```python
from build123d import *

# Parameters (mm, degrees)
F0_R         = 3.95
F0_R_2       = 2.95
F1_DEPTH     = 12
F3_DEPTH     = 4
F5_R         = 5
F6_W         = 3
F6_H         = 7
F6_W_2       = 2.1112600537
F7_DEPTH     = 16.5
F8_W         = 3.25
F8_H         = 1.5
F9_DEPTH     = 7
F10_T1_DEPTH = 34
F10_T3_DEPTH = 24.5


# Not quite as in the source:
# - a fillet or chamfer that OpenCascade refuses, or shapes differently, is made with other operations: its cross-section is extruded or revolved along the edge and cut away or added


with BuildPart() as f1:
    # F0 (on Top) → F1 (new body)
    with BuildSketch(Plane.XY):
        Circle(F0_R)
        Circle(F0_R_2, mode=Mode.SUBTRACT)
    extrude(amount=F1_DEPTH)


with BuildPart() as f1b:
    # F0 (on Top) → F1, piece 2 (new body)
    with BuildSketch(Plane.XY):
        with Locations((29.5, 0)):
            Circle(F0_R)
        with Locations((29.5, 0)):
            Circle(F0_R_2, mode=Mode.SUBTRACT)
    extrude(amount=F1_DEPTH)


with BuildPart() as f3:
    # F2 (on face) → F3 (new body)
    with BuildSketch(Plane(origin=(0, 0, 0), x_dir=(1, 0, 0), z_dir=(0, 0, -1))):
        with BuildLine():
            ThreePointArc((0, 3.95), (2.7930717857, 2.7930717857), (3.95, 0))
            Line((3.95, 0), (25.55, 0))
            ThreePointArc((25.55, 0), (26.7069282143, 2.7930717857), (29.5, 3.95))
            Line((29.5, 3.95), (29.5, 20))
            Line((29.5, 20), (0, 20))
            Line((0, 20), (0, 3.95))
        make_face()
    extrude(amount=-F3_DEPTH)

    # F4: union F1, F1b
    add(f1.part)
    add(f1b.part)

    # F5
    f5_edges = [f3.edges().sort_by_distance(p)[0] for p in [
        (0, -20, 2),
        (29.5, -20, 2),
    ]]
    fillet(f5_edges, radius=F5_R)

    # F6 (on face) → F7 (join)
    with BuildSketch(Plane(origin=(0, 0, 0), x_dir=(1, 0, 0), z_dir=(0, 0, -1))):
        with Locations((-3.6112600537, 11.5)):
            Rectangle(F6_W, F6_H)
        with Locations((-1.0556300269, 11.5)):
            Rectangle(F6_W_2, F6_H)
        with Locations((30.5556300269, 11.5)):
            Rectangle(F6_W_2, F6_H)
        with Locations((33.1112600537, 11.5)):
            Rectangle(F6_W, F6_H)
    extrude(amount=-F7_DEPTH)

    # F8 (on face) → F9 (cut, through all)
    with BuildSketch(Plane.XZ.offset(15)):
        with Locations((-1.625, 12.75)):
            Rectangle(F8_W, F8_H)
        with Locations((31.125, 12.75)):
            Rectangle(F8_W, F8_H)
    extrude(amount=-F9_DEPTH, mode=Mode.SUBTRACT)

    # F10: fillet of radius 3.5 on 6 edges, made by hand

    # F10_s2 → F10_t1 (cut)
    with BuildSketch(Plane.XY.offset(-8.75)):
        with BuildLine():
            ThreePointArc((-1.6112600537, -15), (-4.0861337879, -13.9748737342), (-5.1112600537, -11.5))
            Line((-5.1112600537, -11.5), (-5.1112600537, -15))
            Line((-5.1112600537, -15), (-1.6112600537, -15))
        make_face()
        with BuildLine():
            ThreePointArc((-5.1112600537, -11.5), (-4.0861337879, -9.0251262658), (-1.6112600537, -8))
            Line((-1.6112600537, -8), (-5.1112600537, -8))
            Line((-5.1112600537, -8), (-5.1112600537, -11.5))
        make_face()
        with BuildLine():
            ThreePointArc((34.6112600537, -11.5), (33.5861337879, -13.9748737342), (31.1112600537, -15))
            Line((31.1112600537, -15), (34.6112600537, -15))
            Line((34.6112600537, -15), (34.6112600537, -11.5))
        make_face()
        with BuildLine():
            ThreePointArc((31.1112600537, -8), (33.5861337879, -9.0251262658), (34.6112600537, -11.5))
            Line((34.6112600537, -11.5), (34.6112600537, -8))
            Line((34.6112600537, -8), (31.1112600537, -8))
        make_face()
    extrude(amount=F10_T1_DEPTH, mode=Mode.SUBTRACT)

    # F10_s4 → F10_t3 (cut)
    with BuildSketch(Plane.XZ.offset(-0.75)):
        with BuildLine():
            ThreePointArc((34.6112600537, 13), (33.5861337879, 15.4748737342), (31.1112600537, 16.5))
            Line((31.1112600537, 16.5), (34.6112600537, 16.5))
            Line((34.6112600537, 16.5), (34.6112600537, 13))
        make_face()
        with BuildLine():
            ThreePointArc((-5.1112600537, 13), (-4.0861337879, 15.4748737342), (-1.6112600537, 16.5))
            Line((-1.6112600537, 16.5), (-5.1112600537, 16.5))
            Line((-5.1112600537, 16.5), (-5.1112600537, 13))
        make_face()
    extrude(amount=F10_T3_DEPTH, mode=Mode.SUBTRACT)


solid = f3.part
```
Source: CAD feature listing. Evaluate the final solid. Frame: model axes, mm. A direction names the side the tool comes from. Coordinates: 2 decimals unless noted, no trailing zeros. Write each loop counter-clockwise with the first axis right and the second up, starting at its lowest first coordinate (ties: lowest second). Pieces come first, ordered by that corner, then holes. Notation, with made-up numbers: (5.5, 76.5) - (55.5, 76.5) arc R29 cw to (55.5, 100.5) - close; hole circle Ø11 at (5, 60.25). An arc over 180 degrees is marked (long way). Answer as a JSON object with one key per item and string values.
Q1. Section query D-D, the plane x = 23.5. Output: boundary loops of the cut face in (y, z).
Ans:
{"outline": "(-20, 0) - (0, 0) - (0, 4) - (-20, 4) - close"}
Q2. Section query C-C, the plane y = -9.75. Output: boundary loops of the cut face in (x, z).
Ans:
{"outline": "(-4.64, 0) - (34.14, 0) - (34.14, 14.75) arc R3.5 ccw to (31.11, 16.5) - (29.5, 16.5) - (29.5, 13.5) - (32.75, 13.5) - (32.75, 12) - (29.5, 12) - (29.5, 4) - (0, 4) - (0, 12) - (-3.25, 12) - (-3.25, 13.5) - (0, 13.5) - (0, 16.5) - (-1.61, 16.5) arc R3.5 ccw to (-4.64, 14.75) - close"}
Q3. Draft query along Z for faces 1 (the flat face through (32.75, -12, 13)), 2 (the flat face through (31, -12, 13.5)), 3 (the flat face through (15, -10, 4)), 4 (the flat face through (29.5, -11, 8)). Return one class per face: released by +Z, released by -Z, zero draft, split by the parting line, or undercut.
Ans:
{"face 1": "undercut", "face 2": "undercut", "face 3": "released by +Z", "face 4": "zero draft"}
Q4. Section query B-B, the plane z = 2.25. Output: boundary loops of the cut face in (x, y).
Ans:
{"outline": "(-1.61, -15) - (0, -15) arc R5 ccw to (5, -20) - (24.5, -20) arc R5 ccw to (29.5, -15) - (31.11, -15) arc R3.5 ccw to (31.11, -8) - (29.5, -8) - (29.5, -3.95) arc R3.95 ccw (long way) to (25.55, 0) - (3.95, 0) arc R3.95 ccw (long way) to (0, -3.95) - (0, -8) - (-1.61, -8) arc R3.5 ccw to start; hole circle Ø5.9 at (0, 0); hole circle Ø5.9 at (29.5, 0)"}
Q5. Set-up query: faces 5 (the flat face through (30, -8, 6)), 6 (the flat face through (15, 0, 2)), 7 (the cylindrical face through (-2.91, 2.67, 5.92)). Return all of +Z, -Z, +X, -X, +Y, -Y with unobstructed straight access to the full face (end or side cutting, diameter ignored); none if empty.
Ans:
{"face 5": "+Z, -Z, +X", "face 6": "+Z, -Z, +Y", "face 7": "+Z"}
Q6. Material intervals for line 1 (Y direction, x = -2.5, z = 5); line 2 (X direction, y = -1.25, z = 6.25); line 3 (Y direction, x = -1.5, z = 6.75), sorted ascending. Write a range as [from, to].
Ans:
{"line 1": "y = [-14.89, -8.11], [-3.06, -1.57], [1.57, 3.06]", "line 2": "x = [-3.75, -2.67], [2.67, 3.75], [25.75, 26.83], [32.17, 33.25]", "line 3": "y = [-15, -8], [-3.65, -2.54], [2.54, 3.65]"}
Q7. First-contact query: pin 1 Ø6 at (y, z) = (-7.5, 5.5) entering from +X; pin 2 Ø0.5 at (x, z) = (-0.5, 7.5) entering from +Y; pin 3 Ø8 at (x, y) = (27, -17) entering from -Z; pin 4 Ø5.5 at (x, y) = (0, 0) entering from -Z. Flat tips, straight axial feed; report the tip coordinate or a pass-through.
Ans:
{"pin 1": "stops at x = 34.47", "pin 2": "stops at y = 3.94", "pin 3": "stops at z = 0", "pin 4": "passes through"}
Q8. Section query A-A, the plane z = 9.25. Output: boundary loops of the cut face in (x, y), plus the area to 3 significant figures.
Ans:
{"outline": "circle Ø7.9 at (0, 0); (-1.61, -15) - (0, -15) - (0, -8) - (-1.61, -8) arc R3.5 ccw to start; circle Ø7.9 at (29.5, 0); (29.5, -15) - (31.11, -15) arc R3.5 ccw to (31.11, -8) - (29.5, -8) - close; hole circle Ø5.9 at (0, 0); hole circle Ø5.9 at (29.5, 0)", "area": "104 mm2"}
